```python
from build123d import *

# Parameters (mm, degrees)
SKETCH1_W                      = 75.565
SKETCH1_H                      = 35.56
BOSS_EXTRUDE1_DEPTH            = 3.175
SKETCH6_W                      = 3.175
SKETCH6_H                      = 9.028368652
BOSS_EXTRUDE4_DEPTH            = 14.986
BOSS_EXTRUDE6_DEPTH            = 9.028368652
BOSS_EXTRUDE7_DEPTH            = 75.565
SKETCH10_W                     = 75.565
SKETCH10_H                     = 23.368
BOSS_EXTRUDE8_DEPTH            = 7.545165067
CUT_EXTRUDE1_DEPTH             = 82.438667238
CUT_EXTRUDE2_REACH             = 52.836
SKETCH12_W                     = 6.35
SKETCH12_H                     = 3.175
CUT_EXTRUDE2_DIRECTION_2_DEPTH = 51.836411552
CUT_EXTRUDE3_DEPTH             = 55.765947786
CUT_EXTRUDE4_REACH             = 57.378
SKETCH14_W                     = 2.54
SKETCH14_H                     = 3.81
CUT_EXTRUDE5_REACH             = 57.378
SKETCH15_W                     = 114.661215645
SKETCH15_H                     = 6.578342779


with BuildPart() as part:
    # Sketch1 → Boss-Extrude1 (new body)
    with BuildSketch(Plane.XY):
        Rectangle(SKETCH1_W, SKETCH1_H)
    extrude(amount=-BOSS_EXTRUDE1_DEPTH)

    # Sketch6 → Boss-Extrude4 (add)
    with BuildSketch(Plane.XY):
        with Locations((-36.195, 0)):
            Rectangle(SKETCH6_W, SKETCH6_H)
        with Locations((36.195, 0)):
            Rectangle(SKETCH6_W, SKETCH6_H)
    extrude(amount=BOSS_EXTRUDE4_DEPTH)

    # Sketch8 → Boss-Extrude6 (add)
    with BuildSketch(Plane.XZ.offset(4.514184326)):
        Polygon((-37.7825, 14.986), (-31.4325, 14.986), (-37.7825, 21.336), align=None)
        Polygon((37.7825, 14.986), (31.4325, 14.986), (37.7825, 21.336), align=None)
    extrude(amount=-BOSS_EXTRUDE6_DEPTH)

    # Sketch9 → Boss-Extrude7 (add)
    with BuildSketch(Plane.ZY.offset(37.7825)):
        Polygon((-3.175, 17.78), (-18.572931679, 8.89), (-3.175, -17.78), align=None)
    extrude(amount=-BOSS_EXTRUDE7_DEPTH)

    # Sketch10 → Boss-Extrude8 (add)
    with BuildSketch(Plane(origin=(0, -5.819815329, -10.08021584), x_dir=(-1, 0, 0), z_dir=(0, -0.5000000000000012, -0.8660254037844378))):
        with Locations((0, -2.126431679)):
            Rectangle(SKETCH10_W, SKETCH10_H)
    extrude(amount=BOSS_EXTRUDE8_DEPTH)

    # Sketch11 → Cut-Extrude1 (cut, through all)
    with BuildSketch(Plane.ZY.offset(37.7825)):
        Polygon((-14.859, 2.457281636), (0, 4.514184326), (36.888684706, 18.275511072), (5.286071508, 25.150339228), (-30.3838484, 8.233222823), align=None)
        Polygon((-3.175, -17.78), (-8.125516688, -9.205453573), (0, -4.514184326), (40.158547499, -20.406390647), (15.599703883, -25.394905756), align=None)
    extrude(amount=-CUT_EXTRUDE1_DEPTH, mode=Mode.SUBTRACT)

    # Cut-Extrude2: up to this plane
    cut_extrude2_end = Plane(origin=(37.7825, -9.205453573, -8.125516688), z_dir=(0, 0.8660254037844387, -0.5))
    # Sketch12 → Cut-Extrude2 (cut, up to the surface)
    with BuildSketch(Plane(origin=(0, 4.429308453, -0.61314062), x_dir=(1, 0, 0), z_dir=(0, 0.9905543702216955, -0.13712052958875431)), mode=Mode.PRIVATE) as cut_extrude2_sk1:
        with Locations((0, 4.143512655)):
            Rectangle(SKETCH12_W, SKETCH12_H)
    cut_extrude2_tool1 = split(extrude(cut_extrude2_sk1.sketch, amount=-CUT_EXTRUDE2_REACH, mode=Mode.PRIVATE), bisect_by=cut_extrude2_end, keep=Keep.BOTH, mode=Mode.PRIVATE)
    add(cut_extrude2_tool1.solids().sort_by_distance((0, 3.861148, -4.717515))[0], mode=Mode.SUBTRACT)

    # Sketch12 → Cut-Extrude2 direction 2 (cut)
    with BuildSketch(Plane(origin=(0, 4.429308453, -0.61314062), x_dir=(1, 0, 0), z_dir=(0, 0.9905543702216955, -0.13712052958875431))):
        with Locations((0, 4.143512655)):
            Rectangle(SKETCH12_W, SKETCH12_H)
    extrude(amount=CUT_EXTRUDE2_DIRECTION_2_DEPTH, mode=Mode.SUBTRACT)

    # Sketch13 → Cut-Extrude3 (cut, through all)
    with BuildSketch(Plane(origin=(0, 8.277096964, -4.77878416), x_dir=(1, 0, 0), z_dir=(0, 0.8660254037844379, -0.5000000000000012))):
        Polygon((-31.75, 11.639630657), (-37.7825, 0.917907837), (-37.7825, 11.639630657), (-37.7825, 19.184795724), (-31.75, 19.184795724), align=None)
        Polygon((37.7825, 0.917907837), (37.7825, 11.639630657), (37.7825, 19.184795724), (31.75, 19.184795724), (31.75, 11.639630657), align=None)
    extrude(amount=-CUT_EXTRUDE3_DEPTH, mode=Mode.SUBTRACT)

    # Sketch14 → Cut-Extrude4 (cut, up to next)
    with BuildSketch(Plane(origin=(0, -9.592397862, -16.614520463), x_dir=(-1, 0, 0), z_dir=(0, -0.5000000000000013, -0.8660254037844379)), mode=Mode.PRIVATE) as cut_extrude4_sk1:
        with Locations((-17.78, -6.082892111)):
            Rectangle(SKETCH14_W, SKETCH14_H)
    cut_extrude4_tool1 = extrude(cut_extrude4_sk1.sketch, amount=-CUT_EXTRUDE4_REACH, mode=Mode.PRIVATE) & part.part
    # Sketch14 → Cut-Extrude4 (cut, up to next)
    with BuildSketch(Plane(origin=(0, -9.592397862, -16.614520463), x_dir=(-1, 0, 0), z_dir=(0, -0.5000000000000013, -0.8660254037844379)), mode=Mode.PRIVATE) as cut_extrude4_sk2:
        with Locations((17.78, -6.082892111)):
            Rectangle(SKETCH14_W, SKETCH14_H)
    cut_extrude4_tool2 = extrude(cut_extrude4_sk2.sketch, amount=-CUT_EXTRUDE4_REACH, mode=Mode.PRIVATE) & part.part
    add(cut_extrude4_tool1.solids().sort_by_distance((17.78, -14.860337, -13.573074))[0], mode=Mode.SUBTRACT)
    add(cut_extrude4_tool2.solids().sort_by_distance((-17.78, -14.860337, -13.573074))[0], mode=Mode.SUBTRACT)

    # Sketch15 → Cut-Extrude5 (cut, up to next)
    with BuildSketch(Plane(origin=(0, -9.592397862, -16.614520463), x_dir=(-1, 0, 0), z_dir=(0, -0.5000000000000012, -0.8660254037844378)), mode=Mode.PRIVATE) as cut_extrude5_sk1:
        with Locations((-7.679066914, -12.781603069)):
            Rectangle(SKETCH15_W, SKETCH15_H)
    cut_extrude5_tool1 = extrude(cut_extrude5_sk1.sketch, amount=-CUT_EXTRUDE5_REACH, mode=Mode.PRIVATE) & part.part
    add(cut_extrude5_tool1.solids().sort_by_distance((7.679067, -20.661591, -10.223719))[0], mode=Mode.SUBTRACT)


solid = part.part
```
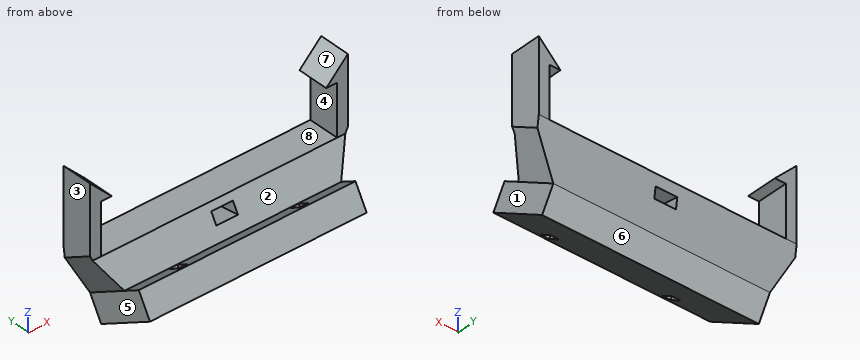
Design review of the part built by this model. Coordinates are the model's own, in mm. Face numbers are marked on the shaded views. A direction names the side the tool comes from. Round coordinates to 2 decimals unless told otherwise and drop trailing zeros. Write each loop counter-clockwise with the first axis right and the second up, starting at its lowest first coordinate (ties: lowest second). Pieces come first, ordered by that corner, then holes.
Item 1: We need section A-A on x = 2. Write out the cut boundary in (y, z), and give its area (3 significant figures).
Item 2: For the marked faces 1, 2, 3 and 4, list the 3-axis set-ups (+Z, -Z, +X, -X, +Y, -Y) from which the entire face can be reached by the end or side of a thin tool; tool diameter is ignored.
Item 3: For probe 1 along X at (y, z) = (-0.25, 1.5); probe 2 along Y at (x, z) = (-30.5, -5.5); probe 3 along X at (y, z) = (1.5, -5) (3 decimals), list the stretches that pass through material, from the lowest coordinate up.
Item 4: The part is to be moulded in two halves that separate along X. For the marked faces 5, 6, 7 and 8, say which applies: +X half, -X half, draft (parallel to the pull), parting line (faces both ways), or undercut.
Item 5: We need section D-D on x = -28. Write out the cut boundary in (y, z).
Item 6: We need section B-B on z = 9.5. Write out the cut boundary in (x, y).
Item 7: Clearance check with flat-ended pins moving along their axes: pin 1 Ø6 at (x, y) = (28, -6) entering from +Z; pin 2 Ø1 at (x, y) = (-23.5, -8) entering from -Z; pin 3 Ø5 at (y, z) = (-1, -4) entering from -X. State where each tip first meets the part, or that it passes through.
Returned:
1. outline: (-17.81, -11.87) - (-1.32, -21.39) - (2.46, -14.86) - (3.64, -6.29) - (-7.27, -4.78) - (-9.21, -8.13) - (-14.04, -5.33) - close; (-5.56, -1.81) - (4.08, -3.15) - (4.51, 0) - (-4.51, 0) - close
1. area: 241 mm2
2. face 1: -Z, +X, -Y
2. face 2: +Z, +X, -X
2. face 3: +Z, -Z, -X, +Y, -Y
2. face 4: +Y, -Y
3. probe 1: x = -37.78 to -34.61, 34.61 to 37.78
3. probe 2: y = -14.14 to -13.75, -7.69 to 3.75
3. probe 3: x = -36.285 to -3.175, 3.175 to 36.285
4. face 5: -X half
4. face 6: draft
4. face 7: undercut
4. face 8: undercut
5. outline: (-17.81, -11.87) - (-1.32, -21.39) - (2.46, -14.86) - (4.51, 0) - (-4.51, 0) - (-9.21, -8.13) - (-14.04, -5.33) - close
6. outline: (-37.78, -4.51) - (-34.61, -4.51) - (-34.61, 4.51) - (-37.78, 4.51) - close; (34.61, -4.51) - (37.78, -4.51) - (37.78, 4.51) - (34.61, 4.51) - close
7. pin 1: stops at z = 0
7. pin 2: stops at z = -17.82
7. pin 3: stops at x = -37.48
